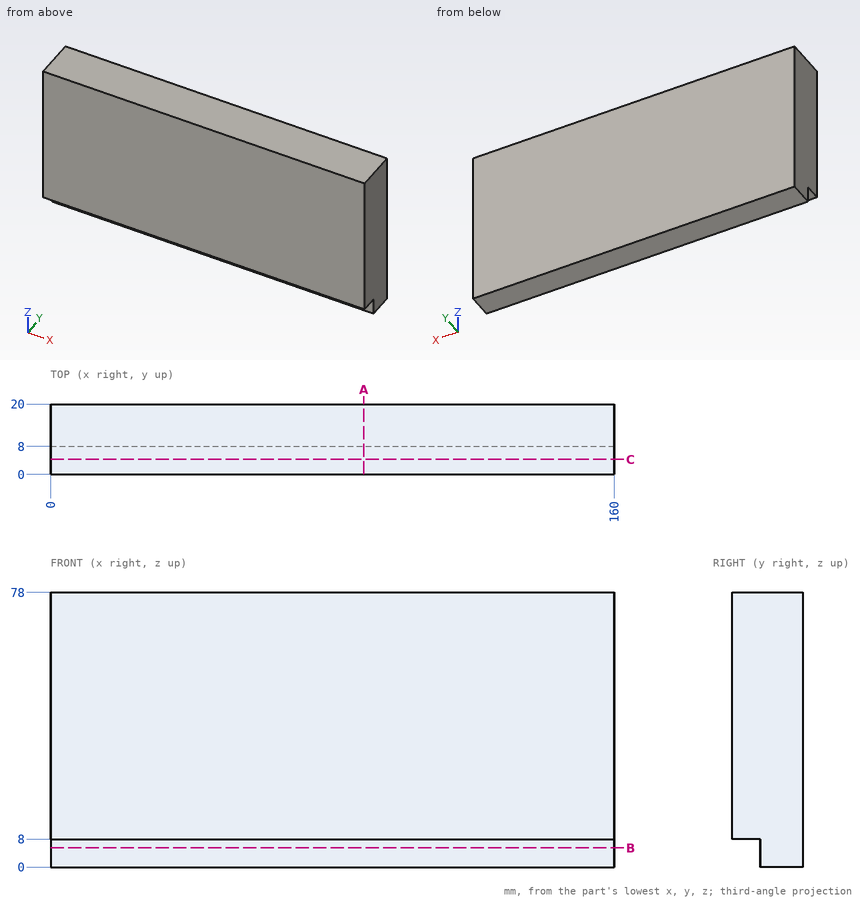
Check sheet for the drawn part. Datum: minimum x, y, z corner. Units: mm. Round coordinates to 2 decimals unless told otherwise and drop trailing zeros. Loops run counter-clockwise (first coordinate to the right, second up) from the corner with the lowest first, then second, coordinate; pieces in that order, holes last. Notation, with made-up numbers: (82.25, 37) -> (104.25, 37) arc R25 ccw to (104.25, 75) -> close; hole circle Ø9 at (37, -5). An arc over 180 degrees is marked (long way). Put each result on its own line as item: value. Start each with the question number.
1. Section check B-B (z = 5.5). Enter the section's corners in (x, y), plus the area to 3 significant figures.
2. Section check A-A (x = 89). Enter the section's corners in (y, z).
3. Section check C-C (y = 4.25). Enter the section's corners in (x, z).
4. Gauge pin test, flat ends, axial feed: pin 1 (9 mm diameter, centred on x = 43, z = 3, fed in from -Y); pin 2 (9 mm diameter, centred on x = 76.5, y = 2.5, fed in from -Z). Record the tip position at first contact, or that the pin passes through.
5. Scan line: probe 1 along Z at (x, y) = (84.5, 4.5). Record every from-to range of solid material in increasing order.
Findings:
1. outline: (0, 8) -> (160, 8) -> (160, 20) -> (0, 20) -> close
1. area: 1,920 mm^2
2. outline: (0, 8) -> (8, 8) -> (8, 0) -> (20, 0) -> (20, 78) -> (0, 78) -> close
3. outline: (0, 8) -> (160, 8) -> (160, 78) -> (0, 78) -> close
4. pin 1: stops at y = 8
4. pin 2: stops at z = 8
5. probe 1: z = 8 to 78
